Build history of the part. All positions in model axes, mm. Coordinates: 2 decimals unless noted, no trailing zeros. Order: outer loops, then holes, each group sorted by start corner. A loop starts at its lowest first (then second) coordinate and runs counter-clockwise, first axis right, second up. Notation, with made-up numbers: (6, -18.75) - (65, -18.75) arc R27 cw to (65, 6.25) - close; hole circle Ø4 at (65.25, -12). An arc over 180 degrees is marked (long way). Write each question's results on one line, items separated by ' | '.
Autodesk Fusion 360 part; units mm, degrees
sketch "Sketch1" plane through (0, 0, 0) normal (0, 0, 1) x (1, 0, 0)
  line L0 (-4.5, 24) -> (4.5, 24)
  line L1 (4.5, 112) -> (-4.5, 112)
  line L2 (-4.5, 112) -> (-4.5, 24)
  line L3 (0, 24) -> (0, 112) construction
  line L4 (4.5, 112) -> (4.5, 24)
  line L5 (0, 24) -> (0, 0) construction
  circle A0 centre (0, 120.9303) radius 10
  dimension "d517" = 9
  dimension "d518" = 88
  dimension "d519" = 24
  dimension "d520" = 20
extrude "Extrude1" add sketch "Sketch1" along normal blind 7 makes body 1
sketch "Sketch2" plane through (0, 0, 0) normal (0, 0, 1) x (1, 0, 0)
  arc A0 (4.5, 112) -> (-4.5, 112) centre (0, 120.9303) ccw construction
  line L0 (4.5, 112) -> (4.5, 24) construction
  line L1 (4.5, 24) -> (-4.5, 24) construction
  line L2 (-4.5, 24) -> (-4.5, 112) construction
  line L3 (4.5, 51.0811) -> (33.1156, 96.8757)
  line L4 (33.1156, 96.8757) -> (43.3486, 90.4815)
  line L5 (43.3486, 90.4815) -> (4.5, 24)
  line L6 (4.5, 24) -> (4.5, 51.0811)
  dimension "d525" = 54
  dimension "d526" = 32
  dimension "d527" = 1.7
  dimension "d528" = 77
extrude "Extrude2" add sketch "Sketch2" along normal up to surface (7 mm away) separate body makes body 2
mirror "Mirror1" about plane through (0, 0, 0) normal (1, 0, 0) of bodies 2 makes body 3
combine "Combine1" operation add target body 2 tool bodies 1 3
sketch "Sketch3" plane through (0, 0, 0) normal (0, 0, 1) x (1, 0, 0)
  line L0 (43.3486, 90.4815) -> (4.5, 24)
  line L1 (4.5, 24) -> (-4.5, 24)
  line L2 (-4.5, 24) -> (-43.3486, 90.4815)
  line L3 (-43.3486, 90.4815) -> (-33.1156, 96.8757)
  line L4 (-33.1156, 96.8757) -> (-4.5, 51.0811)
  line L5 (-4.5, 51.0811) -> (-4.5, 112)
  arc A0 (4.5, 112) -> (-4.5, 112) centre (0, 120.9303) ccw
  line L6 (4.5, 112) -> (4.5, 51.0811)
  line L7 (4.5, 51.0811) -> (33.1156, 96.8757)
  line L8 (33.1156, 96.8757) -> (43.3486, 90.4815)
  line L9 (4.5, 24) -> (6.6025, 11.4359)
  line L10 (6.6025, 11.4359) -> (4.5525, 7.8852)
  line L11 (4.5525, 7.8852) -> (0, 22.1776)
  line L12 (0, 22.1776) -> (-4.5525, 7.8852)
  line L13 (-4.5525, 7.8852) -> (-6.6025, 11.4359)
  line L14 (-6.6025, 11.4359) -> (-4.5, 24)
  line L15 (0, 1.75) -> (0, 22.5)
  line L16 (1.75, 0) -> (22.5, 0)
  dimension "d533" = 60
  dimension "d538" = 15
  dimension "d539" = 4.1
  dimension "d540" = 19
extrude "Extrude3" add sketch "Sketch3" along normal up to surface (7 mm away) separate body contours L1 L9 L10 L11 L12 L13 L14 makes body 4
pattern_circular "C-Pattern1" count 6 over 360 about axis through (0, 0, 1.75) along (0, 0, 1) of bodies 4 makes body 5 at (-14.7812, 12.8073, 0) makes body 6 at (-18.482, -6.3972, 0) makes body 7 at (-3.7008, -19.2045, 0) makes body 8 at (14.7812, -12.8073, 0) makes body 9 at (18.482, 6.3972, 0)
pattern_circular "C-Pattern2" count 6 over 360 about axis through (0, 0, 1.75) along (0, 0, 1) of bodies 2 makes body 10 at (-56.5186, 12.482, 0) makes body 11 at (-39.069, -42.7055, 0) makes body 12 at (17.4495, -55.1875, 0) makes body 13 at (56.5186, -12.482, 0) makes body 14 at (56.5186, 12.482, 0)
combine "Combine2" operation add target body 2 tool bodies 14 13 12 11 10 5 4 9 8 7 6
sketch "Sketch4" plane through (0, 0, 7) normal (0, 0, 1) x (-1, 0, 0)
  arc A0 (-4.5, -112) -> (4.5, -112) centre (0, -120.9303) ccw
  circle A1 centre (0, -120.9303) radius 5
  dimension "d543" = 10
extrude "Extrude4" cut sketch "Sketch4" against normal up to surface (7 mm away) bodies 2
equation "d526 = Angular Dimension-2"
equation "d527 = Angular Dimension-3"
equation "d533 = Angular Dimension-2"
equation "d540 = Angular Dimension-3"
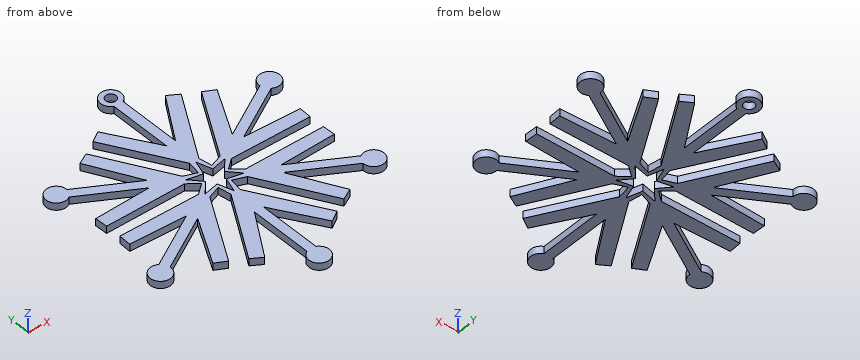
1. Probe line 1 (X direction, y = -83, z = 2.75); line 2 (X direction, y = 88, z = 3); line 3 (X direction, y = -19, z = 4.5). List the from-to ranges inside material, lowest first.
Solved:
line 1: x = -38.98 to -24.45, -4.5 to 4.5, 24.45 to 38.98 | line 2: x = -41.9 to -27.57, -4.5 to 4.5, 27.57 to 41.9 | line 3: x = -100.43 to -20.3, -5.34 to -1.01, 1.01 to 5.34, 20.3 to 100.43
2. Band-saw the part on C-C on z = 3. Give the number of separate pieces and of enclosed holes in the cut face, then the cut area to 3 significant figures.
Solved:
separate pieces: 1 | enclosed holes: 2 | area: 17,400 mm2
3. Band-saw the part on D-D on y = 104.5. Give the cut face in (x, z), then the cut area to 3 significant figures.
Solved:
outline: (-4.5, 0) - (4.5, 0) - (4.5, 7) - (-4.5, 7) - close | area: 63.0 mm2
4. Band-saw the part on B-B on x = 90.5. Give the cut face in (y, z), then the cut area to 3 significant figures.
Solved:
outline: (-57.45, 0) - (-47.05, 0) - (-47.05, 7) - (-57.45, 7) - close; (-20.11, 0) - (-7.75, 0) - (-7.75, 7) - (-20.11, 7) - close; (7.75, 0) - (20.11, 0) - (20.11, 7) - (7.75, 7) - close; (47.05, 0) - (57.45, 0) - (57.45, 7) - (47.05, 7) - close | area: 318 mm2
5. Drop a flat-ended pin along its axis: pin 1 Ø1 at (x, z) = (13, 6) entering from +Y. Give the stop position or say it passes through.
Solved:
pin 1: stops at y = 65.48
6. Band-saw the part on A-A on y = -55.5. Give the cut face in (x, z), then the cut area to 3 significant figures.
Solved:
outline: (-113.41, 0) - (-87.13, 0) - (-87.13, 7) - (-113.41, 7) - close; (-55.85, 0) - (-41.12, 0) - (-41.12, 7) - (-55.85, 7) - close; (-22.91, 0) - (-7.26, 0) - (-7.26, 7) - (-22.91, 7) - close; (-4.5, 0) - (4.5, 0) - (4.5, 7) - (-4.5, 7) - close; (7.26, 0) - (22.91, 0) - (22.91, 7) - (7.26, 7) - close; (41.12, 0) - (55.85, 0) - (55.85, 7) - (41.12, 7) - close; (87.13, 0) - (113.41, 0) - (113.41, 7) - (87.13, 7) - close | area: 856 mm2
